Design review of the part built by this model. Coordinates are the model's own, in mm. Face numbers are marked on the shaded views. A direction names the side the tool comes from. Coordinates: 2 decimals unless noted, no trailing zeros. Write each loop counter-clockwise with the first axis right and the second up, starting at its lowest first coordinate (ties: lowest second). Pieces come first, ordered by that corner, then holes.
Q1. Machinability: for the marked faces 4, 5, 6 and 7, which of the approach directions +Z, -Z, +X, -X, +Y, -Y give a long, thin tool a straight path to every point of the face, cutting with its end or side? Answer none if there is none.
Q2. Add section A-A, the plane y = 252. Give the boundary of the cut face in (x, z).
Q3. Add section C-C, the plane x = 469. Give the boundary of the cut face in (y, z).
Q4. Clearance check with flat-ended pins moving along their axes: pin 1 Ø1 at (x, z) = (261.5, 119.5) entering from -Y; pin 2 Ø3 at (x, y) = (393, 61.5) entering from -Z; pin 3 Ø10 at (x, y) = (158, 121) entering from +Z; pin 4 Ø8 at (y, z) = (260.5, 169.5) entering from -X. State where each tip first meets the part, or that it passes through.
Q5. Add section B-B, the plane z = 19.5. Give the boundary of the cut face in (x, y), plus the area to 3 significant figures.
Q6. Add section D-D, the plane x = 170. Give the boundary of the cut face in (y, z).
Q7. The part is to be moulded in two halves that separate along Y. For the marked faces 1, 2 and 3, say which applies: +Y half, -Y half, draft (parallel to the pull), parting line (faces both ways), or undercut.
Q8. To check wall thickness, follow probe 1 along X at (y, z) = (263.5, 76); probe 2 along X at (y, z) = (211.5, 78.5); probe 3 along X at (y, z) = (139, 43). State the ranges of each line that lie inside material, in increasing order.
from build123d import *

# Parameters (mm, degrees)
BOSS_EXTRUDE1_DEPTH     = 1000
SKETCH2_W               = 100
SKETCH2_H               = 300
BOSS_EXTRUDE2_DEPTH     = 200
SKETCH3_R               = 44.830840268
CUT_EXTRUDE1_DEPTH      = 1
CUT_EXTRUDE1_DEPTH_BACK = 201


with BuildPart() as part:
    # Sketch1 → Boss-Extrude1 (new body)
    with BuildSketch(Plane(origin=(0, 0, 0), x_dir=(0, 0, -1), z_dir=(1, 0, 0))):
        Polygon((0, 0), (-200, 0), (-200, 50), (-100, 300), (0, 50), align=None)
    extrude(amount=BOSS_EXTRUDE1_DEPTH)

    # Sketch2 → Boss-Extrude2 (add)
    with BuildSketch(Plane(origin=(0, 0, 0), x_dir=(-1, 0, 0), z_dir=(0, 0, -1))):
        with Locations((-500, 150)):
            Rectangle(SKETCH2_W, SKETCH2_H)
    extrude(amount=-BOSS_EXTRUDE2_DEPTH)

    # Sketch3 → Cut-Extrude1 (cut, two sides)
    with BuildSketch(Plane(origin=(0, 0, 0), x_dir=(-1, 0, 0), z_dir=(0, 0, -1))) as cut_extrude1_sk:
        with Locations((-503.081055297, 171.556016762)):
            Circle(SKETCH3_R)
    extrude(amount=CUT_EXTRUDE1_DEPTH, mode=Mode.SUBTRACT)
    extrude(cut_extrude1_sk.sketch, amount=-CUT_EXTRUDE1_DEPTH_BACK, mode=Mode.SUBTRACT)


solid = part.part
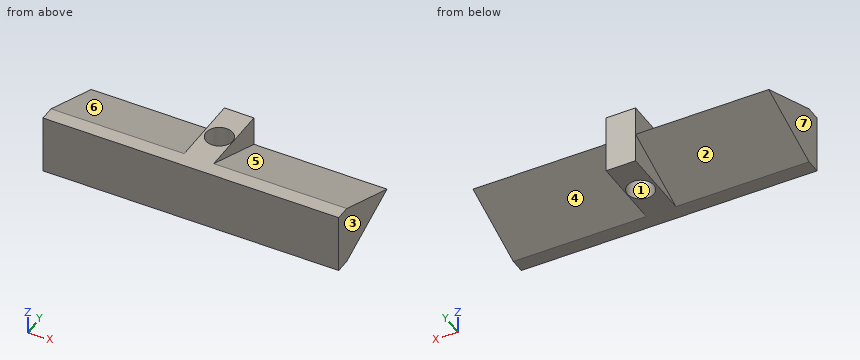
Here are the results:
1. face 4: -Z, +X, +Y
1. face 5: +Z, +X, +Y
1. face 6: +Z, -X, +Y
1. face 7: +Z, -Z, -X, +Y, -Y
2. outline: (0, 80.8) - (450, 80.8) - (450, 0) - (550, 0) - (550, 80.8) - (1000, 80.8) - (1000, 119.2) - (550, 119.2) - (550, 200) - (450, 200) - (450, 119.2) - (0, 119.2) - close
3. outline: (0, 0) - (142.43, 0) - (142.43, 200) - (0, 200) - close; (200.68, 0) - (300, 0) - (300, 200) - (200.68, 200) - close
4. pin 1: stops at y = 0
4. pin 2: stops at z = 4
4. pin 3: stops at z = 173.6
4. pin 4: stops at x = 450
5. outline: (0, 0) - (1000, 0) - (1000, 98.75) - (550, 98.75) - (550, 300) - (450, 300) - (450, 98.75) - (0, 98.75) - close; hole circle Ø89.66 at (503.08, 171.56)
5. area: 113,000 mm2
6. outline: (0, 0) - (50, 0) - (300, 100) - (50, 200) - (0, 200) - close
7. face 1: undercut
7. face 2: +Y half
7. face 3: draft
8. probe 1: x = 450 to 550
8. probe 2: x = 0 to 482.73, 523.43 to 1000
8. probe 3: x = 0 to 472.26, 533.9 to 1000
